The drawing under review shows one solid part. Ordinate dimensions are in mm from its lowest x, y, z. A direction names the side the tool comes from. Coordinates: 2 decimals unless noted, no trailing zeros. Loops run counter-clockwise (first coordinate to the right, second up) from the corner with the lowest first, then second, coordinate; pieces in that order, holes last. Notation, with made-up numbers: M 4.25,3.5 L 9.25,3.5 A13 ccw 9.25,10.5 Z; hole C 89,13 d10. An arc over 180 degrees is marked long. Use one line per item in the form item = value.
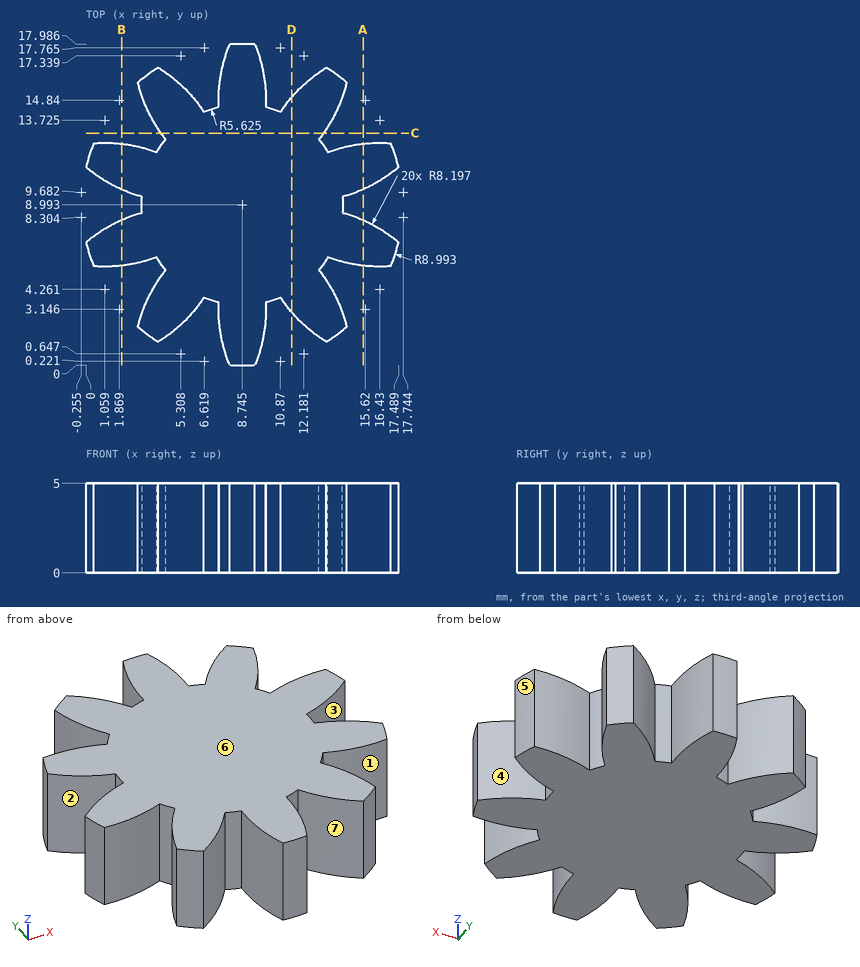
1. Wall thickness on line 1 along X through (y, z) = (15.25, 2.6) (1 decimal); line 2 along Y through (x, z) = (14, 0.4) (1 decimal); line 3 along Y through (x, z) = (3.75, 2.95) (1 decimal): over which ranges is each line inside the solid? List them lowest first. Write a range as from..to.
Computed values:
line_1 = 3.1..5.8, 7.4..10.1, 11.7..14.4
line_2 = 1.7..3.8, 5.9..12.1, 14.2..16.3
line_3 = 1.5..4.3, 6..12, 13.7..16.5
2. Tool access review of the marked faces 1, 2 and 3: name each direction out of +Z, -Z, +X, -X, +Y, -Y from which nothing blocks a thin tool from reaching the whole face with its end or side.
Computed values:
face_1 = +Z, -Z
face_2 = +Z, -Z, -X
face_3 = +Z, -Z, +X
3. For pin 1 Ø1 at (x, z) = (3.5, 1.5) entering from +Y, flat-tipped, find the tip position at first contact; note if it passes through.
Computed values:
pin_1 = 16.63
4. Consider section D-D on x = 11.5. Write out the cut boundary in (y, z).
Computed values:
outline = M 2.99,0 L 14.99,0 L 14.99,5 L 2.99,5 Z
5. Consider section C-C on y = 13. Write out the cut boundary in (x, z).
Computed values:
outline = M 4.2,0 L 13.29,0 L 13.29,5 L 4.2,5 Z
6. Consider section A-A on x = 15.5. Write out the cut boundary in (y, z) (1 decimal), plus the area to 3 significant figures.
Computed values:
outline = M 5.6,0 L 8.1,0 L 8.1,5 L 5.6,5 Z; M 9.8,0 L 12.4,0 L 12.4,5 L 9.8,5 Z
area = 25.6 mm2
7. Draft analysis for pull direction Y (two halves, no side actions). For the marked faces 4, 5, 6 and 7, state which applies: +Y half, -Y half, draft (parallel to the pull), parting line (faces both ways), or undercut.
Computed values:
face_4 = undercut
face_5 = +Y half
face_6 = draft
face_7 = -Y half
